Geometry: final body of the model. Coordinates: model frame, mm. Face numbers are marked on the shaded views. A direction names the side the tool comes from. Coordinates: 2 decimals unless noted, no trailing zeros. Loops run counter-clockwise (first coordinate to the right, second up) from the corner with the lowest first, then second, coordinate; pieces in that order, holes last. Notation, with made-up numbers: (64, -36) - (80, -36) arc R4 ccw to (80, -30) - close; hole circle Ø5 at (16, 29). An arc over 180 degrees is marked (long way). Put each result on its own line as item: value. Start each with the question number.
1) Section C-C on x = -13. Output: boundary loops of the cut face in (y, z), and give its area (3 significant figures).
2) Section D-D on x = -5. Output: boundary loops of the cut face in (y, z), and give its area (3 significant figures).
3) Material intervals for line 1 along Z through (x, y) = (-1, -0.15); line 2 along X through (y, z) = (-1.6, -0.25); line 3 along Z through (x, y) = (16, -0.1), sorted ascending. Write a range as from..to.
4) Contact query for a flat-ended pin moving along its axis: pin 1 Ø1 at (x, y) = (0.5, 0) entering from -Z. Output: stop coordinate, or through.
5) Section A-A on z = 0. Output: boundary loops of the cut face in (x, y).
6) Reachability of the marked faces 1 and 2 from +Z, -Z, +X, -X, +Y, -Y: full face, straight path, thin tool, end or side. Return the list, or none.
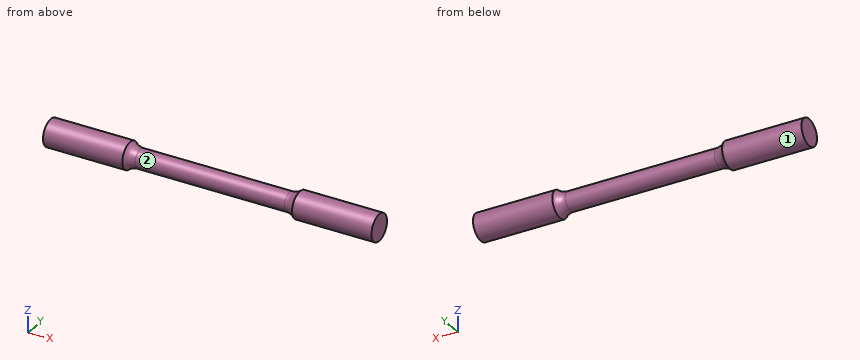
```python
from build123d import *


with BuildPart() as f1:
    # F0 (on Front) → F1 (revolve)
    with BuildSketch(Plane.XZ):
        with BuildLine():
            Line((10, 1.25), (0, 1.25))
            Line((0, 1.25), (-10, 1.25))
            ThreePointArc((-10, 1.25), (-10.737251, 1.390844), (-11.370665, 1.793539))
            Line((-11.370665, 1.793539), (-21.999996, 1.793539))
            Line((-21.999996, 1.793539), (-21.999996, 0))
            Line((-21.999996, 0), (0, 0))
            Line((0, 0), (21.999996, 0))
            Line((21.999996, 0), (21.999996, 1.793539))
            Line((21.999996, 1.793539), (11.370665, 1.793539))
            ThreePointArc((11.370665, 1.793539), (10.737251, 1.390844), (10, 1.25))
        make_face()
    revolve(axis=Axis((-10.999998, 0, 0), (1, 0, 0)))


solid = f1.part
```
Answer block:
1. outline: circle Ø3.59 at (0, 0)
1. area: 10.1 mm²
2. outline: circle Ø2.5 at (0, 0)
2. area: 4.91 mm²
3. line 1: z = -1.24..1.24
3. line 2: x = -22..-11.16, 11.16..22
3. line 3: z = -1.79..1.79
4. pin 1: stops at z = -1.25
5. outline: (-22, -1.79) - (-11.37, -1.79) arc R2 cw to (-10, -1.25) - (10, -1.25) arc R2 cw to (11.37, -1.79) - (22, -1.79) - (22, 1.79) - (11.37, 1.79) arc R2 cw to (10, 1.25) - (-10, 1.25) arc R2 cw to (-11.37, 1.79) - (-22, 1.79) - close
6. face 1: +X, -X
6. face 2: none
